CAD build for the part. Positions are in the model's coordinates, mm. Face numbers are marked on the shaded views. A direction names the side the tool comes from. Coordinates: 2 decimals unless noted, no trailing zeros. Loops run counter-clockwise (first coordinate to the right, second up) from the corner with the lowest first, then second, coordinate; pieces in that order, holes last. Notation, with made-up numbers: (11, 27.5) -> (61, 27.5) arc R22 ccw to (61, 63.5) -> close; hole circle Ø8 at (51.25, 14). An arc over 180 degrees is marked (long way). Write each question's results on one line, items separated by ' | '.
```python
from build123d import *

# Parameters (mm, degrees)
BOX001_W          = 23
BOX001_H          = 6
BOX001_DEPTH      = 10
BOX002_W          = 6
BOX002_H          = 23
BOX002_DEPTH      = 10
CYLINDER001_R     = 10.45
CYLINDER001_DEPTH = 100
CYLINDER_R        = 12.6
CYLINDER_DEPTH    = 34
BOX_W             = 10
BOX_H             = 3.6
BOX_DEPTH         = 34


with BuildPart() as cube:
    # Box001 → Box001 (new body)
    with BuildSketch(Plane(origin=(-11.5, -3, 0), x_dir=(1, 0, 0), z_dir=(0, 0, 1))):
        with Locations((11.5, 3)):
            Rectangle(BOX001_W, BOX001_H)
    extrude(amount=BOX001_DEPTH)


with BuildPart() as cube001:
    # Box002 → Box002 (new body)
    with BuildSketch(Plane(origin=(-3, -11.5, 0), x_dir=(1, 0, 0), z_dir=(0, 0, 1))):
        with Locations((3, 11.5)):
            Rectangle(BOX002_W, BOX002_H)
    extrude(amount=BOX002_DEPTH)


with BuildPart() as cylinder:
    # Cylinder001 → Cylinder001 (new body)
    with BuildSketch(Plane.XY):
        Circle(CYLINDER001_R)
    extrude(amount=CYLINDER001_DEPTH)


with BuildPart() as outside:
    # Cylinder → Cylinder (new body)
    with BuildSketch(Plane.XY):
        Circle(CYLINDER_R)
    extrude(amount=CYLINDER_DEPTH)


with BuildPart() as final:
    # Box → Box (new body)
    with BuildSketch(Plane(origin=(6, -1.8, 0), x_dir=(1, 0, 0), z_dir=(0, 0, 1))):
        with Locations((5, 1.8)):
            Rectangle(BOX_W, BOX_H)
    extrude(amount=BOX_DEPTH)

    # Fusion: union Outside
    add(outside.part)

    # Cut: cut Cylinder
    add(cylinder.part, mode=Mode.SUBTRACT)

    # Cut001: cut Cube001
    add(cube001.part, mode=Mode.SUBTRACT)

    # Cut002: cut Cube
    add(cube.part, mode=Mode.SUBTRACT)


solid = final.part
```
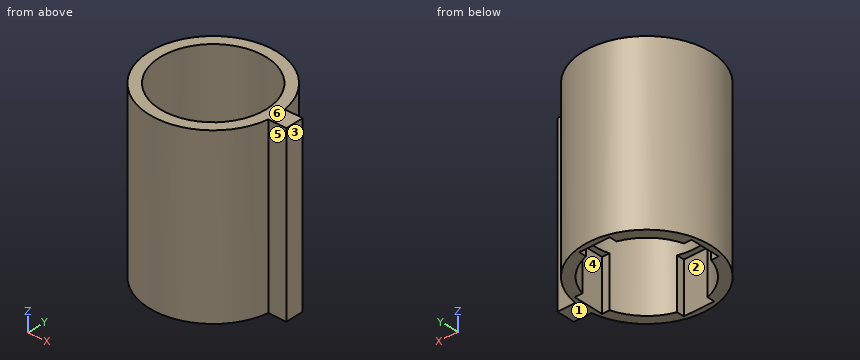
Q1. Drop flat-ended pins along their axis: pin 1 (5 mm diameter, centred on y = 9, z = 23, fed in from +X); pin 2 (3 mm diameter, centred on y = 8.5, z = 15, fed in from -X); pin 3 (1.8 mm diameter, centred on x = -0.5, z = 5, fed in from +Y); pin 4 (5 mm diameter, centred on y = 6.5, z = 14.5, fed in from -X). Give the stop position or say it passes through.
Results are:
pin 1: x = 10.79 | pin 2: x = -10.48 | pin 3: y = 12.6 | pin 4: x = -11.95
Q2. Pull direction X, two halves, no side cores. Call the marked faces 1, 2 and 3: +X half, -X half, draft (parallel to the pull), parting line (faces both ways), or undercut.
Results are:
face 1: draft | face 2: undercut | face 3: +X half
Q3. Cut at C-C on z = 26. Write the cut outline in (x, y).
Results are:
outline: (12.47, -1.8) -> (16, -1.8) -> (16, 1.8) -> (12.47, 1.8) arc R12.6 ccw (long way) to start; hole circle Ø20.9 at (0, 0)
Q4. Which spindle directions (+Z, -Z, +X, -X, +Y, -Y) get a long thin tool onto all of the face, cutting with end or side? Do the marked faces 4, 5 and 6. Say none if no direction does.
Results are:
face 4: -Z | face 5: +Z, -Z, +X, -Y | face 6: +Z, +X, -X, +Y, -Y
Q5. Cut at B-B on y = 0. Write the cut outline in (x, z).
Results are:
outline: (-12.6, 0) -> (-11.5, 0) -> (-11.5, 10) -> (-10.45, 10) -> (-10.45, 34) -> (-12.6, 34) -> close; (10.45, 10) -> (11.5, 10) -> (11.5, 0) -> (16, 0) -> (16, 34) -> (10.45, 34) -> close
Q6. Cut at D-D on y = -9.5. Write the cut outline in (x, z), and give its area (3 significant figures).
Results are:
outline: (-8.28, 0) -> (-4.35, 0) -> (-4.35, 34) -> (-8.28, 34) -> close; (4.35, 0) -> (8.28, 0) -> (8.28, 34) -> (4.35, 34) -> close | area: 267 mm^2
Q7. Cut at A-A on x = 0. Write the cut outline in (y, z).
Results are:
outline: (-12.6, 0) -> (-11.5, 0) -> (-11.5, 10) -> (-10.45, 10) -> (-10.45, 34) -> (-12.6, 34) -> close; (10.45, 10) -> (11.5, 10) -> (11.5, 0) -> (12.6, 0) -> (12.6, 34) -> (10.45, 34) -> close
Q8. Wall check: L1, parallel to Y at x = 0, z = 27.5; L2, parallel to Y at x = 0, z = 8.5; L3, parallel to X at y = -3.25, z = 31. Give the ranges that are in metal, low to high. Write a range as from..to.
Results are:
L1: -12.6..-10.45, 10.45..12.6 | L2: -12.6..-11.5, 11.5..12.6 | L3: -12.17..-9.93, 9.93..12.17
